```python
from build123d import *

# Parameters (mm, degrees)
ESQUISSE1_W             = 60
ESQUISSE1_H             = 100
BOSS_EXTRU_1_DEPTH      = 10
ESQUISSE2_W             = 30
ESQUISSE2_H             = 10
BOSS_EXTRU_2_DEPTH      = 60
ESQUISSE3_W             = 60
ESQUISSE3_H             = 10
BOSS_EXTRU_3_DEPTH      = 70
BOSS_EXTRU_4_DEPTH      = 9
ESQUISSE6_R             = 4
ENL_V_MAT_EXTRU_2_DEPTH = 142.421356237
CONG_1_R                = 10


with BuildPart() as part:
    # Esquisse1 → Boss.-Extru.1 (new body)
    with BuildSketch(Plane(origin=(0, 0, 0), x_dir=(1, 0, 0), z_dir=(0, 1, 0))):
        with Locations((30, 50)):
            Rectangle(ESQUISSE1_W, ESQUISSE1_H)
    extrude(amount=BOSS_EXTRU_1_DEPTH)

    # Esquisse2 → Boss.-Extru.2 (add)
    with BuildSketch(Plane(origin=(0, 10, 0), x_dir=(1, 0, 0), z_dir=(0, 1, 0))):
        with Locations((45, 5)):
            Rectangle(ESQUISSE2_W, ESQUISSE2_H)
    extrude(amount=BOSS_EXTRU_2_DEPTH)

    # Esquisse3 → Boss.-Extru.3 (add)
    with BuildSketch(Plane(origin=(0, 10, 0), x_dir=(1, 0, 0), z_dir=(0, 1, 0))):
        with Locations((30, 95)):
            Rectangle(ESQUISSE3_W, ESQUISSE3_H)
    extrude(amount=BOSS_EXTRU_3_DEPTH)

    # Esquisse8 → Boss.-Extru.4 (add)
    with BuildSketch(Plane(origin=(0, 10, 0), x_dir=(1, 0, 0), z_dir=(0, 1, 0))):
        Polygon((0, 0), (0, 55), (40, 55), (40, 10), (30, 10), (30, 0), align=None)
    extrude(amount=BOSS_EXTRU_4_DEPTH)

    # Esquisse6 → Enlèv. mat.-Extru.2 (cut, through all)
    with BuildSketch(Plane(origin=(0, 0, -100), x_dir=(-1, 0, 0), z_dir=(0, 0, -1))):
        with Locations((-45, 40)):
            Circle(ESQUISSE6_R)
        with Locations((-13, 64)):
            Circle(ESQUISSE6_R)
    extrude(amount=-ENL_V_MAT_EXTRU_2_DEPTH, mode=Mode.SUBTRACT)

    # Congé1
    cong_1_edges = [part.edges().sort_by_distance(p)[0] for p in [
        (0, 80, -95),
        (60, 80, -95),
        (30, 70, -5),
        (60, 70, -5),
    ]]
    fillet(cong_1_edges, radius=CONG_1_R)


solid = part.part
```
For this review, take the finished solid that the model builds, in its own axes (mm). A direction names the side the tool comes from. Coordinates: 2 decimals unless noted, no trailing zeros. Write each loop counter-clockwise with the first axis right and the second up, starting at its lowest first coordinate (ties: lowest second). Pieces come first, ordered by that corner, then holes. Notation, with made-up numbers: (16, 67.25) -> (66, 67.25) arc R17 cw to (66, 95.25) -> close; hole circle Ø11 at (14.25, 81). An arc over 180 degrees is marked (long way). Put each result on its own line as item: value.
Q1. Wall thickness on L1, parallel to Z at x = 51.5, y = 49.5; L2, parallel to Y at x = 45, z = -98; L3, parallel to Y at x = 13, z = -93: over which ranges is each line inside the solid? List them lowest first.
From the geometry:
L1: z = -100 to -90, -10 to 0
L2: y = 0 to 36, 44 to 80
L3: y = 0 to 60, 68 to 80
Q2. Take a section at D-D, the plane z = -53.5. State the section outline as (x, y) points, then the cut area to 3 significant figures.
From the geometry:
outline: (0, 0) -> (60, 0) -> (60, 10) -> (40, 10) -> (40, 19) -> (0, 19) -> close
area: 960 mm2
Q3. Take a section at A-A, the plane x = 45. State the section outline as (y, z) points, then the cut area to 3 significant figures.
From the geometry:
outline: (0, -100) -> (36, -100) -> (36, -90) -> (10, -90) -> (10, -10) -> (36, -10) -> (36, 0) -> (0, 0) -> close; (44, -100) -> (80, -100) -> (80, -90) -> (44, -90) -> close; (44, -10) -> (70, -10) -> (70, 0) -> (44, 0) -> close
area: 2,140 mm2
Q4. Clearance check with flat-ended pins moving along their axes: pin 1 Ø10 at (x, z) = (48, -18.5) entering from +Y; pin 2 Ø11 at (y, z) = (45, -7) entering from -X; pin 3 Ø1.5 at (x, z) = (17.5, -38) entering from -Y; pin 4 Ø20 at (x, z) = (12, -40) entering from +Y. State where each tip first meets the part, or that it passes through.
From the geometry:
pin 1: stops at y = 10
pin 2: stops at x = 30
pin 3: stops at y = 0
pin 4: stops at y = 19
Q5. Tool access review of faces 4 (the flat face through (45, 70, -5)), 5 (the cylindrical face through (57.15, 66.99, -5.07)), 6 (the flat face through (30, 45, -90)), 7 (the cylindrical face through (32.85, 66.99, -5.07)), 8 (the flat face through (0, 14, -53)): name each direction out of +Z, -Z, +X, -X, +Y, -Y from which nothing blocks a thin tool from reaching the whole face with its end or side.
From the geometry:
face 4: +Z, +X, -X, +Y
face 5: +Z, +X, +Y
face 6: +X, -X, +Y
face 7: +Z, -X, +Y
face 8: +Z, -Z, -X, +Y, -Y
Q6. Take a section at B-B, the plane y = 40. State the section outline as (x, z) points, then the cut area to 3 significant figures.
From the geometry:
outline: (0, -100) -> (41, -100) -> (41, -90) -> (0, -90) -> close; (30, -10) -> (41, -10) -> (41, 0) -> (30, 0) -> close; (49, -100) -> (60, -100) -> (60, -90) -> (49, -90) -> close; (49, -10) -> (60, -10) -> (60, 0) -> (49, 0) -> close
area: 740 mm2
Q7. Take a section at C-C, the plane y = 25. State the section outline as (x, z) points, then the cut area to 3 significant figures.
From the geometry:
outline: (0, -100) -> (60, -100) -> (60, -90) -> (0, -90) -> close; (30, -10) -> (60, -10) -> (60, 0) -> (30, 0) -> close
area: 900 mm2
Q8. The part is to be moulded in two halves that separate along Z. For faces 1 (the flat face through (40, 14, -33)), 2 (the flat face through (30, 39, -5)), 3 (the flat face through (37, 27, 0)), say which applies: +Z half, -Z half, draft (parallel to the pull), parting line (faces both ways), or undercut.
From the geometry:
face 1: undercut
face 2: draft
face 3: +Z half
